The listing builds one solid part. Answer for the finished solid, in the listing's coordinates (mm). Face numbers are marked on the shaded views. A direction names the side the tool comes from. Coordinates: 2 decimals unless noted, no trailing zeros. Write each loop counter-clockwise with the first axis right and the second up, starting at its lowest first coordinate (ties: lowest second). Pieces come first, ordered by that corner, then holes. Notation, with made-up numbers: M 47.5,-33.5 L 105.5,-33.5 A35 cw 105.5,3.5 Z; hole C 37.5,26 d3. An arc over 180 degrees is marked long. Answer as CSV lines item,"result". Start each with the question number.
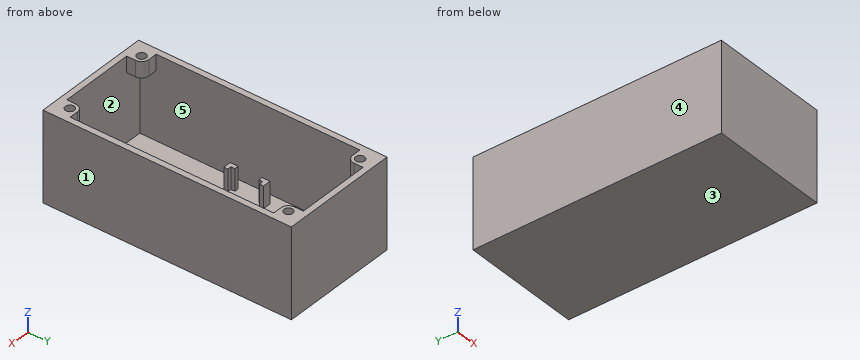
```python
from build123d import *

# Parameters (mm, degrees)
SKETCH_W        = 60
SKETCH_H        = 125
PAD_DEPTH       = 45
SKETCH001_W     = 54
SKETCH001_H     = 119
POCKET_DEPTH    = 42
PAD001_DEPTH    = 8
SKETCH003_R     = 2.25
POCKET001_DEPTH = 7
PAD002_DEPTH    = 11


with BuildPart() as part:
    # Sketch → Pad (new body)
    with BuildSketch(Plane.XY):
        Rectangle(SKETCH_W, SKETCH_H)
    extrude(amount=PAD_DEPTH)

    # Sketch001 (on Face6 of Pad) → Pocket (cut)
    with BuildSketch(Plane.XY.offset(45)):
        Rectangle(SKETCH001_W, SKETCH001_H)
    extrude(amount=-POCKET_DEPTH, mode=Mode.SUBTRACT)

    # Sketch002 (on Face5 of Pocket) → Pad001 (join)
    with BuildSketch(Plane.XY.offset(45)):
        with BuildLine():
            ThreePointArc((22.5, -51.25), (19.84835, -52.34835), (18.75, -55))
            Line((18.75, -60.445518), (18.75, -55))
            Line((18.75, -60.445518), (27, -59.5))
            Line((27.750854, -51.25), (27, -59.5))
            Line((27.750854, -51.25), (22.5, -51.25))
        make_face()
        with BuildLine():
            Line((-18.75, -60.445518), (-27, -59.5))
            Line((-27.750854, -51.25), (-27, -59.5))
            Line((-27.750854, -51.25), (-22.5, -51.25))
            ThreePointArc((-18.75, -55), (-19.84835, -52.34835), (-22.5, -51.25))
            Line((-18.75, -60.445518), (-18.75, -55))
        make_face()
        with BuildLine():
            Line((-18.75, 60.445518), (-27, 59.5))
            Line((-27.750854, 51.25), (-27, 59.5))
            Line((-27.750854, 51.25), (-22.5, 51.25))
            ThreePointArc((-22.5, 51.25), (-19.84835, 52.34835), (-18.75, 55))
            Line((-18.75, 60.445518), (-18.75, 55))
        make_face()
        with BuildLine():
            Line((18.75, 60.445518), (18.75, 55))
            ThreePointArc((18.75, 55), (19.84835, 52.34835), (22.5, 51.25))
            Line((27.750854, 51.25), (22.5, 51.25))
            Line((27.750854, 51.25), (27, 59.5))
            Line((18.75, 60.445518), (27, 59.5))
        make_face()
    extrude(amount=-PAD001_DEPTH)

    # Sketch003 (on Face6 of Pad001) → Pocket001 (cut)
    with BuildSketch(Plane.XY.offset(45)):
        with Locations((22.5, 55)):
            Circle(SKETCH003_R)
        with Locations((-22.5, 55)):
            Circle(SKETCH003_R)
        with Locations((22.5, -55)):
            Circle(SKETCH003_R)
        with Locations((-22.5, -55)):
            Circle(SKETCH003_R)
    extrude(amount=-POCKET001_DEPTH, mode=Mode.SUBTRACT)

    # Sketch004 (on Face32 of Pocket001) → Pad002 (join)
    with BuildSketch(Plane.XY.offset(3)):
        Polygon((-18, 8), (-18, 10), (-22, 10), (-22, 6), (-20, 6), (-20, 8), align=None)
        Polygon((-18, -8), (-18, -10), (-22, -10), (-22, -6), (-20, -6), (-20, -8), align=None)
        Polygon((22, 8), (22, 10), (26, 10), (26, 6), (24, 6), (24, 8), align=None)
        Polygon((22, -8), (22, -10), (26, -10), (26, -6), (24, -6), (24, -8), align=None)
    extrude(amount=PAD002_DEPTH)


solid = part.part
```
1) The part is cut by section B-B (x = -5). Determine the outline of the cut face in (y, z), then the cut area to 3 significant figures.
2) The part is cut by section A-A (z = 18). Determine the outline of the cut face in (x, y).
3) Which of the six approach directions +Z, -Z, +X, -X, +Y, -Y give full straight-line access (tool end or side, diameter ignored) to the marked faces 4 and 5?
4) The part is cut by section C-C (y = -4). Determine the outline of the cut face in (x, z).
5) Each of these flat-tipped pins is pushed along its axis until it touches: P1, Ø2, axis at x = 23.5, y = -7.5, coming from the +Z side; P2, Ø3, axis at x = 10.5, y = 9.5, coming from the +Z side. Where does it stop, or does it pass through?
6) Find the intervals of material crossed by line 1 (Y direction, x = -22.5, z = 42.75); line 2 (X direction, y = -54, z = 34.5), in increasing order. Write a range as from..to.
7) For a pull along Z with two mould halves and no side action, classify the marked faces 1, 2 and 3 as +Z half, -Z half, draft (parallel to the pull), parting line (faces both ways), or undercut.
Completed:
1,outline,"M -62.5,0 L 62.5,0 L 62.5,45 L 59.5,45 L 59.5,3 L -59.5,3 L -59.5,45 L -62.5,45 Z"
1,area,"627 mm²"
2,outline,"M -30,-62.5 L 30,-62.5 L 30,62.5 L -30,62.5 Z; hole M -27,-59.5 L 27,-59.5 L 27,59.5 L -27,59.5 Z"
3,face 4,"+Z, -Z, -X, +Y, -Y"
3,face 5,"none"
4,outline,"M -30,0 L 30,0 L 30,45 L 27,45 L 27,3 L -27,3 L -27,45 L -30,45 Z"
5,P1,"z = 14"
5,P2,"z = 3"
6,line 1,"-62.5..-57.25, -52.75..-51.25, 51.25..52.75, 57.25..62.5"
6,line 2,"-30..-27, 27..30"
7,face 1,"draft"
7,face 2,"undercut"
7,face 3,"-Z half"
